from build123d import *

# Parameters (mm, degrees)
CHAMFER1_SIZE           = 0.5
FILLET1_R               = 0.2
CUT_EXTRUDE1_DEPTH      = 43.775694052
CUT_EXTRUDE1_DEPTH_BACK = 5
FILLET2_R               = 0.2


with BuildPart() as part:
    # Sketch1 → Revolve1 (revolve)
    with BuildSketch(Plane.YZ, mode=Mode.PRIVATE) as revolve1_sk:
        Polygon((0, 36.4), (2, 36.4), (2, 0), (4, 0), (4, -6), (0, -6), align=None)
    revolve(revolve1_sk.sketch.rotate(Axis((0, 0, 38.548402149), (0, 0, -1)), 90), axis=Axis((0, 0, 38.548402149), (0, 0, -1)))

    # Chamfer1
    chamfer1_edges = [part.edges().sort_by_distance(p)[0] for p in [
        (-2, 0, 36.4),
    ]]
    chamfer(chamfer1_edges, length=CHAMFER1_SIZE)

    # Fillet1
    fillet1_edges = [part.edges().sort_by_distance(p)[0] for p in [
        (-4, 0, -6),
        (-4, 0, 0),
    ]]
    fillet(fillet1_edges, radius=FILLET1_R)

    # Sketch2 → Cut-Extrude1 (cut, two sides: drawn at the far end of the back side and taken through both)
    with BuildSketch(Plane(origin=(0, 0, -6), x_dir=(1, 0, 0), z_dir=(0, 0, -1)).offset(-CUT_EXTRUDE1_DEPTH_BACK)):
        Polygon((0, -3), (2.598076211, -1.5), (2.598076211, 1.5), (0, 3), (-2.598076211, 1.5), (-2.598076211, -1.5), align=None)
    extrude(amount=CUT_EXTRUDE1_DEPTH + CUT_EXTRUDE1_DEPTH_BACK, mode=Mode.SUBTRACT)

    # Fillet2
    fillet2_edges = [part.edges().sort_by_distance(p)[0] for p in [
        (-2.598076211, 1.5, -3.5),
        (-1.299038106, 2.25, -1),
        (0, 3, -3.5),
        (1.299038106, 2.25, -1),
        (2.598076211, 1.5, -3.5),
        (2.598076211, 0, -1),
        (2.598076211, -1.5, -3.5),
        (1.299038106, -2.25, -1),
        (0, -3, -3.5),
        (-1.299038106, -2.25, -1),
        (-2.598076211, -1.5, -3.5),
        (-2.598076211, 0, -1),
        (-1.299038106, 2.25, -6),
        (1.299038106, 2.25, -6),
        (2.598076211, 0, -6),
        (1.299038106, -2.25, -6),
        (-1.299038106, -2.25, -6),
        (-2.598076211, 0, -6),
    ]]
    fillet(fillet2_edges, radius=FILLET2_R)


solid = part.part
Input: part model. Units: mm. Frame: model coordinates. A direction names the side the tool comes from. Coordinates: 2 decimals unless noted, no trailing zeros. Loops run counter-clockwise (first coordinate to the right, second up) from the corner with the lowest first, then second, coordinate; pieces in that order, holes last.
Q1. Material intervals for line 1 (Z direction, x = 0, y = 2.75); line 2 (Y direction, x = -1.25, z = -3.5); line 3 (Z direction, x = -0.5, y = 1), sorted ascending.
Q2. Draft query along X for faces 4 (the face through (0, 2, 18)), 5 (the face through (0, 0, 36.4)), 6 (the face through (1.29, 2.19, -1.06)). Return one class per face: +X half, -X half, draft (parallel to the pull), parting line (faces both ways), or undercut.
Q3. Set-up query: faces 1 (the face through (-1.31, -2.31, -5.94)), 2 (the face through (-3, 0, -6)), 3 (the face through (-2, 2, 0)). Return all of +Z, -Z, +X, -X, +Y, -Y with unobstructed straight access to the full face (end or side cutting, diameter ignored); none if empty.
Q4. Cut plane A-A (y = 0). Output: boundary loops of the cut face in (x, z).
Q5. Cut plane B-B (z = 10.5). Output: boundary loops of the cut face in (x, y).
Q6. Contact query for a flat-ended pin moving along its axis: pin 1 (1.5 mm diameter, centred on x = 1.5, y = 1, fed in from -Z). Output: stop coordinate, or through.
Working result:
1. line 1: z = -1 to 0
1. line 2: y = -3.8 to -2.28, 2.28 to 3.8
1. line 3: z = -1 to 36.4
2. face 4: parting line
2. face 5: draft
2. face 6: undercut
3. face 1: -Z
3. face 2: -Z, +X, -X, +Y, -Y
3. face 3: +Z
4. outline: (-4, -5.8) arc R0.2 ccw to (-3.8, -6) - (-2.8, -6) arc R0.2 ccw to (-2.6, -5.8) - (-2.6, -1.2) arc R0.2 cw to (-2.4, -1) - (2.4, -1) arc R0.2 cw to (2.6, -1.2) - (2.6, -5.8) arc R0.2 ccw to (2.8, -6) - (3.8, -6) arc R0.2 ccw to (4, -5.8) - (4, -0.2) arc R0.2 ccw to (3.8, 0) - (2, 0) - (2, 35.9) - (1.5, 36.4) - (-1.5, 36.4) - (-2, 35.9) - (-2, 0) - (-3.8, 0) arc R0.2 ccw to (-4, -0.2) - close
5. outline: circle Ø4 at (0, 0)
6. pin 1: stops at z = -1
